from build123d import *

# Parameters (mm, degrees)
SKETCH1_R           = 1.5
SKETCH1_R_2         = 33
BOSS_EXTRUDE1_DEPTH = 2
CUT_EXTRUDE1_DEPTH  = 74.566296631
FILLET1_R           = 1


with BuildPart() as part:
    # Sketch1 → Boss-Extrude1 (new body)
    with BuildSketch(Plane(origin=(0, 0, 0), x_dir=(1, 0, 0), z_dir=(0, 1, 0))):
        with BuildLine():
            Line((17.897079586, 48.929734976), (40.149284407, 43.651218265))
            ThreePointArc((40.149284407, 43.651218265), (42.540265174, 42.312242187), (43.866371506, 39.91409958))
            Line((43.866371506, 39.91409958), (49.02521675, 17.633846579))
            ThreePointArc((49.02521675, 17.633846579), (49.23478351, 16.809026698), (49.479249782, 15.993868858))
            ThreePointArc((49.479249782, 15.993868858), (51.999812242, -0.139738387), (49.392575566, -16.259565766))
            ThreePointArc((49.392575566, -16.259565766), (49.143731732, -17.073397941), (48.929734976, -17.897079586))
            Line((48.929734976, -17.897079586), (43.651218265, -40.149284407))
            ThreePointArc((43.651218265, -40.149284407), (42.312242187, -42.540265174), (39.91409958, -43.866371506))
            Line((39.91409958, -43.866371506), (17.633846579, -49.02521675))
            ThreePointArc((17.633846579, -49.02521675), (16.809026698, -49.23478351), (15.993868858, -49.479249782))
            ThreePointArc((15.993868858, -49.479249782), (-0.139738387, -51.999812242), (-16.259565766, -49.392575566))
            ThreePointArc((-16.259565766, -49.392575566), (-17.073397941, -49.143731732), (-17.897079586, -48.929734976))
            Line((-17.897079586, -48.929734976), (-40.149284407, -43.651218265))
            ThreePointArc((-40.149284407, -43.651218265), (-42.540265174, -42.312242187), (-43.866371506, -39.91409958))
            Line((-43.866371506, -39.91409958), (-49.02521675, -17.633846579))
            ThreePointArc((-49.02521675, -17.633846579), (-49.23478351, -16.809026698), (-49.479249782, -15.993868858))
            ThreePointArc((-49.479249782, -15.993868858), (-51.999812242, 0.139738387), (-49.392575566, 16.259565766))
            ThreePointArc((-49.392575566, 16.259565766), (-49.143731732, 17.073397941), (-48.929734976, 17.897079586))
            Line((-48.929734976, 17.897079586), (-43.651218265, 40.149284407))
            ThreePointArc((-43.651218265, 40.149284407), (-42.312242187, 42.540265174), (-39.91409958, 43.866371506))
            Line((-39.91409958, 43.866371506), (-17.633846579, 49.02521675))
            ThreePointArc((-17.633846579, 49.02521675), (-16.809026698, 49.23478351), (-15.993868858, 49.479249782))
            ThreePointArc((-15.993868858, 49.479249782), (-8.026622704, 51.3767781), (0.139738387, 51.999812242))
            ThreePointArc((0.139738387, 51.999812242), (8.302633013, 51.332896714), (16.259565766, 49.392575566))
            ThreePointArc((16.259565766, 49.392575566), (17.073397941, 49.143731732), (17.897079586, 48.929734976))
        make_face()
        with Locations(Location((-38.8907, 38.8907, 0), (0, 0, 270))):
            Circle(SKETCH1_R, mode=Mode.SUBTRACT)
        with Locations(Location((38.8907, 38.8907, 0), (0, 0, 90))):
            Circle(SKETCH1_R, mode=Mode.SUBTRACT)
        with Locations(Location((38.8907, -38.8907, 0), (0, 0, 270))):
            Circle(SKETCH1_R, mode=Mode.SUBTRACT)
        with Locations(Location((-38.8907, -38.8907, 0), (0, 0, 90))):
            Circle(SKETCH1_R, mode=Mode.SUBTRACT)
        with Locations(Location((0, 0, 0), (0, 0, 270))):
            Circle(SKETCH1_R_2, mode=Mode.SUBTRACT)
        with Locations(Location((-32.475952642, 18.75, 0), (0, 0, 270))):
            Circle(SKETCH1_R, mode=Mode.SUBTRACT)
        with Locations(Location((0, -37.5, 0), (0, 0, 270))):
            Circle(SKETCH1_R, mode=Mode.SUBTRACT)
        with Locations(Location((32.475952642, 18.75, 0), (0, 0, 270))):
            Circle(SKETCH1_R, mode=Mode.SUBTRACT)
    extrude(amount=BOSS_EXTRUDE1_DEPTH)

    # Sketch2 → Cut-Extrude1 (cut, through all)
    with BuildSketch(Plane(origin=(0, 2, 0), x_dir=(1, 0, 0), z_dir=(0, 1, 0))):
        with BuildLine():
            Line((-8.541028488, 31.875552268), (-10.999809417, 41.051847617))
            ThreePointArc((-10.999809417, 41.051847617), (0, 42.5), (10.999809417, 41.051847617))
            Line((10.999809417, 41.051847617), (8.541028488, 31.875552268))
            ThreePointArc((8.541028488, 31.875552268), (0, 33), (-8.541028488, 31.875552268))
        make_face()
        with BuildLine():
            Line((-31.875552268, -8.541028488), (-41.051847617, -10.999809417))
            ThreePointArc((-41.051847617, -10.999809417), (-36.806079661, -21.25), (-30.0520382, -30.0520382))
            Line((-30.0520382, -30.0520382), (-23.334523779, -23.334523779))
            ThreePointArc((-23.334523779, -23.334523779), (-28.578838325, -16.5), (-31.875552268, -8.541028488))
        make_face()
        with BuildLine():
            Line((23.334523779, -23.334523779), (30.0520382, -30.0520382))
            ThreePointArc((30.0520382, -30.0520382), (36.806079661, -21.25), (41.051847617, -10.999809417))
            Line((41.051847617, -10.999809417), (31.875552268, -8.541028488))
            ThreePointArc((31.875552268, -8.541028488), (28.578838325, -16.5), (23.334523779, -23.334523779))
        make_face()
    extrude(amount=-CUT_EXTRUDE1_DEPTH, mode=Mode.SUBTRACT)

    # Fillet1
    fillet1_edges = [part.edges().sort_by_distance(p)[0] for p in [
        (8.541028488, 1, -31.875552268),
        (-8.541028488, 1, -31.875552268),
        (-10.999809417, 1, -41.051847617),
        (10.999809417, 1, -41.051847617),
        (-31.875552268, 1, 8.541028488),
        (-23.334523779, 1, 23.334523779),
        (-30.0520382, 1, 30.0520382),
        (-41.051847617, 1, 10.999809417),
        (23.334523779, 1, 23.334523779),
        (31.875552268, 1, 8.541028488),
        (41.051847617, 1, 10.999809417),
        (30.0520382, 1, 30.0520382),
    ]]
    fillet(fillet1_edges, radius=FILLET1_R)


solid = part.part
Could you check a few things on this model? Use its own coordinates, in mm. A direction names the side the tool comes from. Give positions to 0.01 mm unless a question says otherwise; leave off trailing zeros. Loops run counter-clockwise (first coordinate to the right, second up) from the corner with the lowest first, then second, coordinate; pieces in that order, holes last. Notation, with made-up numbers: (20.5, -37) -> (32.5, -37) arc R11 cw to (32.5, -25) -> close; hole circle Ø3 at (21.5, -8). An arc over 180 degrees is marked (long way). Answer as CSV lines item,"result". Start each with the question number.
(1) If we section it at B-B on y = 0.3: Count the separate pieces of the cut face and the enclosed holes in it, then the cut area to 3 significant figures.
(2) We'd pull the mould along Z, two halves only. Please class faces 1 (the flat face through (-46.327, 0.986, -28.867)), 2 (the cylindrical face through (-36.877, 1.014, 21.127)), 3 (the cylindrical face through (42.34, 0.99, 42.51)): released by +Z, released by -Z, zero draft, split by the parting line, or undercut.
(3) If we section it at A-A on z = -30: Write out the boundary of the cut face in (x, y), then the cut area to 3 significant figures.
(4) Which directions (+Z, -Z, +X, -X, +Y, -Y) give clear straight access to the entire face, cutting with the end or side of a thin tool? Please do faces 4 (the cylindrical face through (0, 1, 33)), 5 (the cylindrical face through (-42.34, 0.99, -42.51)).
(5) If we section it at C-C on z = 34.5: Write out the boundary of the cut face in (x, y), then the cut area to 3 significant figures.
(6) I need wall thicknesses on probe 1 along X at (y, z) = (1.2, -38.5); probe 2 along X at (y, z) = (1.35, 29.5); probe 3 along X at (y, z) = (0.35, -10). Which ranges of each line are inside material? Lowest first, please.
Computed:
1,separate pieces,"1"
1,enclosed holes,"8"
1,area,"5,100 mm2"
2,face 1,"released by -Z"
2,face 2,"undercut"
2,face 3,"released by +Z"
3,outline,"(-46.06, 0) -> (-13.75, 0) -> (-13.75, 2) -> (-46.06, 2) -> close; (13.75, 0) -> (46.16, 0) -> (46.16, 2) -> (13.75, 2) -> close"
3,area,"129 mm2"
4,face 4,"+Y, -Y"
4,face 5,"-Z, -X, +Y, -Y"
5,outline,"(-45.12, 0) -> (44.99, 0) -> (44.99, 2) -> (-45.12, 2) -> close"
5,area,"180 mm2"
6,probe 1,"x = -44.04 to -40.34, -37.44 to -10.32, 10.32 to 37.44, 40.34 to 44.19"
6,probe 2,"x = -46.28 to -30.54, -29.55 to -14.79, 14.79 to 29.55, 30.54 to 46.18"
6,probe 3,"x = -51.03 to -31.45, 31.45 to 51.03"
